Here's how the part is built. I have some questions about the finished solid (model axes, mm). Face numbers are marked on the shaded views. Coordinates: 2 decimals unless noted, no trailing zeros. Write each loop counter-clockwise with the first axis right and the second up, starting at its lowest first coordinate (ties: lowest second). Pieces come first, ordered by that corner, then holes. Notation, with made-up numbers: (58, -18.75) - (93, -18.75) arc R12 cw to (93, 1.25) - close; hole circle Ø8 at (37, 10). An arc over 180 degrees is marked (long way). Answer in a Markdown table with one row per item. Add a question column.
Item 1: Imagine slicing it at A-A (z = 0). Please give me the cut outline in (x, y), plus the area to 3 significant figures.
Item 2: Imagine slicing it at D-D (x = -6). Please give me the cut outline in (y, z).
Item 3: Imagine slicing it at C-C (x = -26.97). Please give me the cut outline in (y, z).
Item 4: I'm going to push flat-ended pins straight in: pin 1 (5 mm diameter, centred on x = -6.5, y = -7.5, fed in from +Z); pin 2 (3 mm diameter, centred on x = 36.5, y = -9, fed in from -Z); pin 3 (2 mm diameter, centred on x = 36, y = 4.5, fed in from +Z). Where does each tip first touch, or does it pass through?
Item 5: If I drill on probe 1 along X at (y, z) = (1, 0); probe 2 along X at (y, z) = (1.5, 0.75); probe 3 along Z at (x, y) = (26, -3.5), over which ranges is the centre line in solid material (lowest first)? Write a range as from..to.
Item 6: We'd pull the mould along Z, two halves only. Please class the marked faces 1, 2 and 3: +Z half, -Z half, draft (parallel to the pull), parting line (faces both ways), or undercut.
Item 7: Imagine slicing it at B-B (y = 0). Please give me the cut outline in (x, z), plus the area to 3 significant figures.
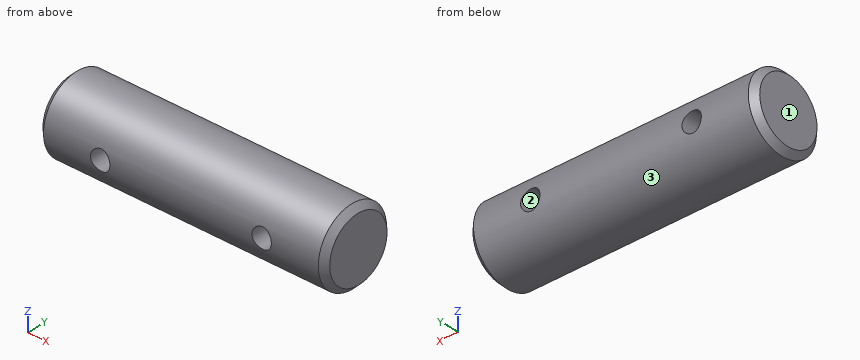
from build123d import *

# Parameters (mm, degrees)
ESBO_O1_R                  = 12.5
RESSALTO_EXTRUS_O1_DEPTH   = 47.91
CHANFRO1_SIZE              = 2
CORTE_EXTRUS_O1_DEPTH      = 52.067289922
CORTE_EXTRUS_O1_DEPTH_BACK = 52.067289922
ESBO_O2_R                  = 3.25


with BuildPart() as part:
    # Esboço1 → Ressalto-extrusão1 (new, symmetric)
    with BuildSketch(Plane(origin=(0, 0, 0), x_dir=(0, -1, 0), z_dir=(1, 0, 0))):
        with Locations(Location((0, 0, 0), (0, 0, 90))):
            Circle(ESBO_O1_R)
    extrude(amount=RESSALTO_EXTRUS_O1_DEPTH, both=True)

    # Chanfro1
    chanfro1_edges = [part.edges().sort_by_distance(p)[0] for p in [
        (-47.91, 0, 12.5),
        (47.91, 0, 12.5),
    ]]
    chamfer(chanfro1_edges, length=CHANFRO1_SIZE)

    # Esboço2 → Corte-extrusão1 (cut, two sides: drawn at the far end of the back side and taken through both)
    with BuildSketch(Plane(origin=(0, 0, 0), x_dir=(1, 0, 0), z_dir=(0, 1, 0)).offset(-CORTE_EXTRUS_O1_DEPTH_BACK)):
        with Locations(Location((-26.97, 0, 0), (0, 0, 270))):
            Circle(ESBO_O2_R)
        with Locations(Location((26.97, 0, 0), (0, 0, 270))):
            Circle(ESBO_O2_R)
    extrude(amount=CORTE_EXTRUS_O1_DEPTH + CORTE_EXTRUS_O1_DEPTH_BACK, mode=Mode.SUBTRACT)


solid = part.part
Here are the results:
| question | item | result |
|---|---|---|
| 1 | outline | (-47.91, -10.5) - (-45.91, -12.5) - (-30.22, -12.5) - (-30.22, 12.5) - (-45.91, 12.5) - (-47.91, 10.5) - close; (-23.72, -12.5) - (23.72, -12.5) - (23.72, 12.5) - (-23.72, 12.5) - close; (30.22, -12.5) - (45.91, -12.5) - (47.91, -10.5) - (47.91, 10.5) - (45.91, 12.5) - (30.22, 12.5) - close |
| 1 | area | 2,060 mm2 |
| 2 | outline | circle Ø25 at (0, 0) |
| 3 | outline | (-12.07, -3.25) arc R12.5 ccw to (12.07, -3.25) - close; (-12.07, 3.25) - (12.07, 3.25) arc R12.5 ccw to start |
| 4 | pin 1 | stops at z = 11.46 |
| 4 | pin 2 | stops at z = -10 |
| 4 | pin 3 | stops at z = 12 |
| 5 | probe 1 | x = -47.91..-30.22, -23.72..23.72, 30.22..47.91 |
| 5 | probe 2 | x = -47.91..-30.13, -23.81..23.81, 30.13..47.91 |
| 5 | probe 3 | z = -12..-3.1, 3.1..12 |
| 6 | face 1 | draft |
| 6 | face 2 | undercut |
| 6 | face 3 | parting line |
| 7 | outline | (-47.91, -10.5) - (-45.91, -12.5) - (45.91, -12.5) - (47.91, -10.5) - (47.91, 10.5) - (45.91, 12.5) - (-45.91, 12.5) - (-47.91, 10.5) - close; hole circle Ø6.5 at (-26.97, 0); hole circle Ø6.5 at (26.97, 0) |
| 7 | area | 2,320 mm2 |
